Part model, mm, in its own coordinate system. A direction names the side the tool comes from. Give positions to 0.01 mm unless a question says otherwise; leave off trailing zeros. Order: outer loops, then holes, each group sorted by start corner. A loop starts at its lowest first (then second) coordinate and runs counter-clockwise, first axis right, second up.
1. Probe line 1 (X direction, y = 25.8, z = -4.5); line 2 (Y direction, x = 52.5, z = 2.1); line 3 (Y direction, x = 24, z = 4.5). List the from-to ranges inside material, lowest first.
2. Slice it at C-C on y = 12.75. List the corners of the cut face in (x, z).
3. Drop flat-ended pins along their axis: pin 1 Ø4 at (x, y) = (7.5, 12.75) entering from +Z; pin 2 Ø14 at (x, y) = (38, 8) entering from -Z; pin 3 Ø7.5 at (x, z) = (22.5, 6) entering from +Y; pin 4 Ø6 at (x, z) = (36.5, -5) entering from -Y. Give the stop position or say it passes through.
4. Slice it at A-A on x = 50. List the corners of the cut face in (y, z).
5. Slice it at B-B on z = -4.5. List the corners of the cut face in (x, y), and give its area (3 significant figures).
6. Slice it at D-D on x = 22. List the corners of the cut face in (y, z), and give its area (3 significant figures).
7. Mould opens along Y. For faces 1 (the cylindrical face through (8.536, 26.521, -4.825)), 2 (the flat face through (30, -3, 5)), 3 (the cylindrical face through (6.579, 13.595, 1.479)) say: +Y half, -Y half, draft (parallel to the pull), parting line (faces both ways), or undercut.
8. Which spindle directions (+Z, -Z, +X, -X, +Y, -Y) get a long thin tool onto all of the face, cutting with end or side? Do faces 4 (the cylindrical face through (53.7, 13.1, 1.5)), 5 (the flat face through (30, 0, 7)), 6 (the flat face through (30, 11, 0)). Say none if no direction does.
from build123d import *

# Parameters (mm, degrees)
SKETCH1_W           = 60
SKETCH1_H           = 25
SKETCH1_R           = 1.25
BOSS_EXTRUDE1_DEPTH = 3
SKETCH2_W           = 60
SKETCH2_H           = 10
BOSS_EXTRUDE2_DEPTH = 3
SKETCH3_W           = 60
SKETCH3_H           = 15
BOSS_EXTRUDE3_DEPTH = 3
SKETCH4_R           = 1.5
CUT_EXTRUDE1_DEPTH  = 3


with BuildPart() as part:
    # Sketch1 → Boss-Extrude1 (new body)
    with BuildSketch(Plane.XY):
        with Locations((30, 12.5)):
            Rectangle(SKETCH1_W, SKETCH1_H)
        with Locations((7.5, 12.75)):
            Circle(SKETCH1_R, mode=Mode.SUBTRACT)
        with Locations((52.5, 12.75)):
            Circle(SKETCH1_R, mode=Mode.SUBTRACT)
    extrude(amount=BOSS_EXTRUDE1_DEPTH)

    # Sketch2 → Boss-Extrude2 (add)
    with BuildSketch(Plane.XZ):
        with Locations((30, 5)):
            Rectangle(SKETCH2_W, SKETCH2_H)
    extrude(amount=BOSS_EXTRUDE2_DEPTH)

    # Sketch3 → Boss-Extrude3 (add)
    with BuildSketch(Plane(origin=(0, 25, 0), x_dir=(1, 0, 0), z_dir=(0, 1, 0))):
        with Locations((30, 4.5)):
            Rectangle(SKETCH3_W, SKETCH3_H)
    extrude(amount=BOSS_EXTRUDE3_DEPTH)

    # Sketch4 → Cut-Extrude1 (cut)
    with BuildSketch(Plane(origin=(0, 28, 0), x_dir=(1, 0, 0), z_dir=(0, 1, 0))):
        with Locations(Location((10, 4.5, 0), (0, 0, 270))):
            Circle(SKETCH4_R)
        with Locations(Location((50, 4.5, 0), (0, 0, 270))):
            Circle(SKETCH4_R)
    extrude(amount=-CUT_EXTRUDE1_DEPTH, mode=Mode.SUBTRACT)


solid = part.part
Data:
1. line 1: x = 0 to 8.5, 11.5 to 48.5, 51.5 to 60
1. line 2: y = -3 to 11.5, 14 to 28
1. line 3: y = -3 to 0
2. outline: (0, 0) - (6.25, 0) - (6.25, 3) - (0, 3) - close; (8.75, 0) - (51.25, 0) - (51.25, 3) - (8.75, 3) - close; (53.75, 0) - (60, 0) - (60, 3) - (53.75, 3) - close
3. pin 1: stops at z = 3
3. pin 2: stops at z = 0
3. pin 3: stops at y = 28
3. pin 4: stops at y = 25
4. outline: (-3, 0) - (25, 0) - (25, -3) - (28, -3) - (28, 3) - (0, 3) - (0, 10) - (-3, 10) - close; (25, -12) - (28, -12) - (28, -6) - (25, -6) - close
5. outline: (0, 25) - (8.5, 25) - (8.5, 28) - (0, 28) - close; (11.5, 25) - (48.5, 25) - (48.5, 28) - (11.5, 28) - close; (51.5, 25) - (60, 25) - (60, 28) - (51.5, 28) - close
5. area: 162 mm2
6. outline: (-3, 0) - (25, 0) - (25, -12) - (28, -12) - (28, 3) - (0, 3) - (0, 10) - (-3, 10) - close
6. area: 150 mm2
7. face 1: draft
7. face 2: -Y half
7. face 3: undercut
8. face 4: +Z, -Z
8. face 5: +Z, +X, -X, +Y
8. face 6: -Z, +X, -X, -Y
